The figure shows three views and two pictorial views of one solid part (mm, origin at its lowest corner). Answer the questions. Coordinates: 2 decimals unless noted, no trailing zeros. Write each loop counter-clockwise with the first axis right and the second up, starting at its lowest first coordinate (ties: lowest second). Pieces come first, ordered by that corner, then holes.
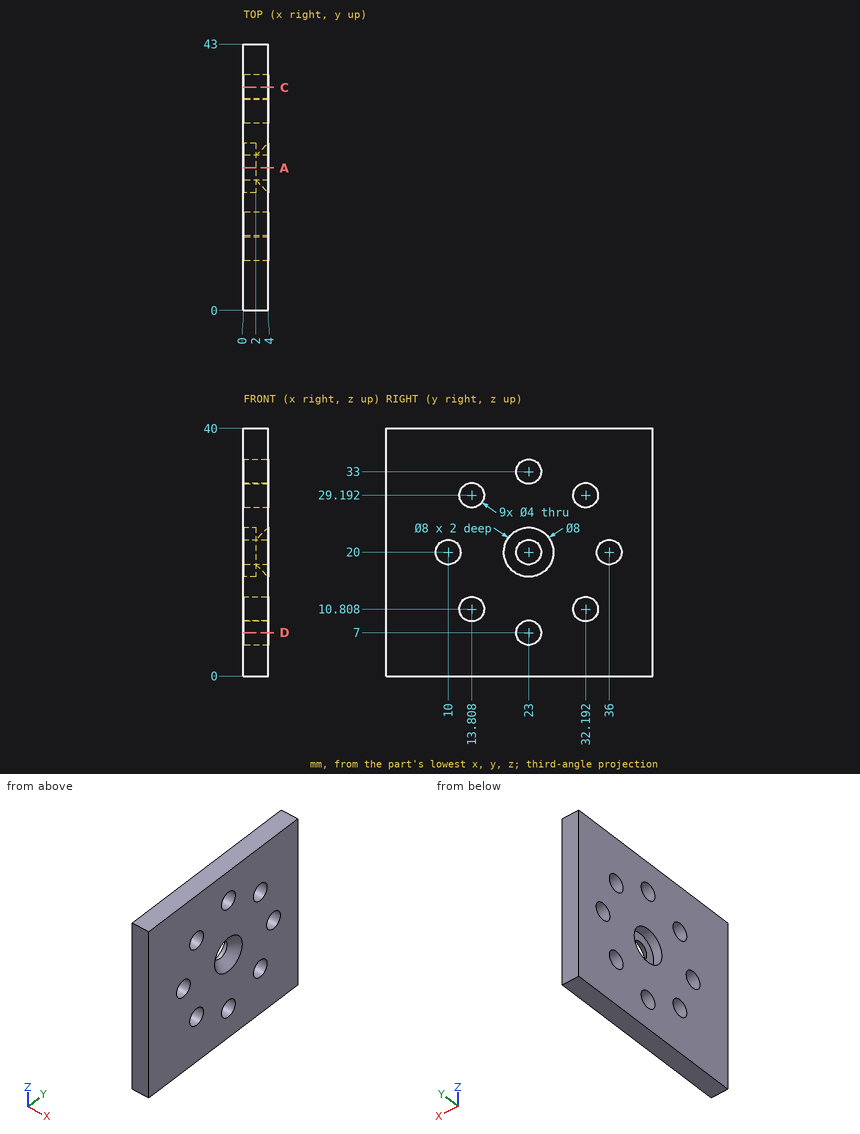
Q1. The part is cut by section C-C, the plane y = 36. Write down the section's boundary in (x, z), then the cut area to 3 significant figures.
Answers below:
outline: (0, 0) - (4, 0) - (4, 18) - (0, 18) - close; (0, 22) - (4, 22) - (4, 40) - (0, 40) - close
area: 144 mm2
Q2. Given pin 1 (2.5 mm diameter, centred on y = 13.81, z = 29.19, fed in from +X); pin 2 (4.5 mm diameter, centred on y = 23, z = 20, fed in from -X), each flat-ended and moving along its own axis, determine where each tip first touches the part or whether it passes through.
Answers below:
pin 1: passes through
pin 2: stops at x = 2
Q3. Find the intervals of material crossed by probe 1 along Z at (x, y) = (0.85, 14); probe 2 along Z at (x, y) = (0.5, 23.5); probe 3 along Y at (x, z) = (0.8, 20), in increasing order.
Answers below:
probe 1: z = 0 to 8.82, 12.8 to 27.2, 31.18 to 40
probe 2: z = 0 to 5.06, 8.94 to 16.03, 23.97 to 31.06, 34.94 to 40
probe 3: y = 0 to 8, 12 to 19, 27 to 34, 38 to 43
Q4. The part is cut by section A-A, the plane y = 23. State how many separate pieces and enclosed holes the cut face has, then the cut area to 3 significant figures.
Answers below:
separate pieces: 4
enclosed holes: 0
area: 100 mm2
Q5. The part is cut by section D-D, the plane z = 7. Write down the section's boundary in (x, y).
Answers below:
outline: (0, 0) - (4, 0) - (4, 21) - (0, 21) - close; (0, 25) - (4, 25) - (4, 43) - (0, 43) - close
